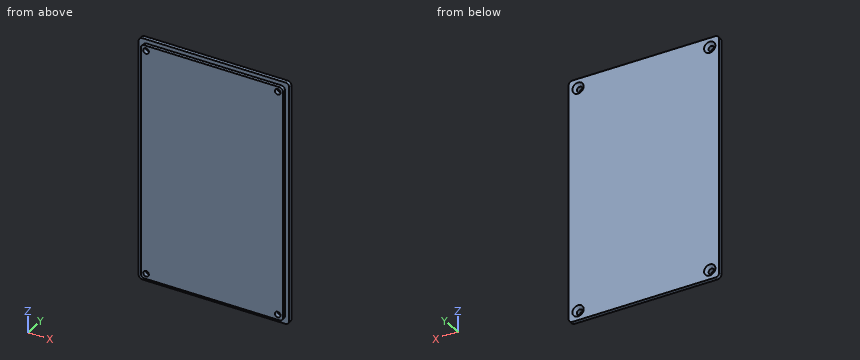
```python
from build123d import *

# Parameters (mm, degrees)
SKETCH1_W           = 75.6
SKETCH1_H           = 125.6
BOSS_EXTRUDE1_DEPTH = 1.8
SKETCH2_W           = 80
SKETCH2_H           = 130
BOSS_EXTRUDE2_DEPTH = 2
SKETCH3_R           = 1.5
CUT_EXTRUDE1_DEPTH  = 77.416228643
CHAMFER1_SIZE       = 1.5
FILLET1_R           = 2


with BuildPart() as part:
    # Sketch1 → Boss-Extrude1 (new body)
    with BuildSketch(Plane(origin=(0, 0, 0), x_dir=(1, 0, 0), z_dir=(0, 1, 0))):
        Rectangle(SKETCH1_W, SKETCH1_H)
    extrude(amount=BOSS_EXTRUDE1_DEPTH)

    # Sketch2 → Boss-Extrude2 (add)
    with BuildSketch(Plane(origin=(0, 1.8, 0), x_dir=(1, 0, 0), z_dir=(0, 1, 0))):
        Rectangle(SKETCH2_W, SKETCH2_H)
    extrude(amount=BOSS_EXTRUDE2_DEPTH)

    # Sketch3 → Cut-Extrude1 (cut, through all)
    with BuildSketch(Plane(origin=(0, 3.8, 0), x_dir=(1, 0, 0), z_dir=(0, 1, 0))):
        with Locations(Location((-35, 60, 0), (0, 0, 270))):
            Circle(SKETCH3_R)
        with Locations(Location((35, 60, 0), (0, 0, 270))):
            Circle(SKETCH3_R)
        with Locations(Location((35, -60, 0), (0, 0, 270))):
            Circle(SKETCH3_R)
        with Locations(Location((-35, -60, 0), (0, 0, 270))):
            Circle(SKETCH3_R)
    extrude(amount=-CUT_EXTRUDE1_DEPTH, mode=Mode.SUBTRACT)

    # Chamfer1
    chamfer1_edges = [part.edges().sort_by_distance(p)[0] for p in [
        (-35, 3.8, 58.5),
        (35, 3.8, 58.5),
        (35, 3.8, -61.5),
        (-35, 3.8, -61.5),
    ]]
    chamfer(chamfer1_edges, length=CHAMFER1_SIZE)

    # Fillet1
    fillet1_edges = [part.edges().sort_by_distance(p)[0] for p in [
        (40, 2.8, 65),
        (40, 2.8, -65),
        (-40, 2.8, -65),
        (-40, 2.8, 65),
        (37.8, 0.9, 62.8),
        (-37.8, 0.9, 62.8),
        (-37.8, 0.9, -62.8),
        (37.8, 0.9, -62.8),
    ]]
    fillet(fillet1_edges, radius=FILLET1_R)


solid = part.part
```
Read the model definition and answer for the solid it produces. Units are mm, in the model's axes. Give positions to 0.01 mm unless a question says otherwise; leave off trailing zeros. Order: outer loops, then holes, each group sorted by start corner. A loop starts at its lowest first (then second) coordinate and runs counter-clockwise, first axis right, second up. Notation, with made-up numbers: (36.25, -33) -> (62.25, -33) arc R25 ccw to (62.25, -17) -> close; hole circle Ø8 at (14, 56.25). An arc over 180 degrees is marked (long way). Write item = value, one per line.
1. A cutting plane is placed at A-A, the plane y = 0.7. Write down the section's boundary in (x, z), and give its area (3 significant figures).
Numbers:
outline = (-37.8, -60.8) arc R2 ccw to (-35.8, -62.8) -> (35.8, -62.8) arc R2 ccw to (37.8, -60.8) -> (37.8, 60.8) arc R2 ccw to (35.8, 62.8) -> (-35.8, 62.8) arc R2 ccw to (-37.8, 60.8) -> close; hole circle Ø3 at (-35, -60); hole circle Ø3 at (-35, 60); hole circle Ø3 at (35, -60); hole circle Ø3 at (35, 60)
area = 9,460 mm²
2. Given pin 1 (0.5 mm diameter, centred on y = 0.5, z = 17, fed in from +X); pin 2 (2 mm diameter, centred on y = 0.5, z = -6, fed in from -X); pin 3 (0.5 mm diameter, centred on x = 4.5, y = 0.5, fed in from +Z), each flat-ended and moving along its own axis, determine where each tip first touches the part or whether it passes through.
Numbers:
pin_1 = 37.8
pin_2 = -37.8
pin_3 = 62.8
3. A cutting plane is placed at C-C, the plane z = -9.5. Write down the section's boundary in (x, y).
Numbers:
outline = (-40, 1.8) -> (-37.8, 1.8) -> (-37.8, 0) -> (37.8, 0) -> (37.8, 1.8) -> (40, 1.8) -> (40, 3.8) -> (-40, 3.8) -> close
4. Straight lines are drawn through the part: line 1 along X through (y, z) = (1.3, 60); line 2 along Z through (x, y) = (35.5, 1.7); line 3 along X through (y, z) = (1.4, -28.5). For each, find the intervals that lie inside material, in ascending order.
Numbers:
line_1 = -37.8 to -36.5, -33.5 to 33.5, 36.5 to 37.8
line_2 = -62.8 to -61.41, -58.59 to 58.59, 61.41 to 62.8
line_3 = -37.8 to 37.8
5. A cutting plane is placed at B-B, the plane x = -23. Write down the section's boundary in (y, z).
Numbers:
outline = (0, -62.8) -> (1.8, -62.8) -> (1.8, -65) -> (3.8, -65) -> (3.8, 65) -> (1.8, 65) -> (1.8, 62.8) -> (0, 62.8) -> close
